Geometry: final body of the model. Coordinates: model frame, mm. A direction names the side the tool comes from. Give positions to 0.01 mm unless a question says otherwise; leave off trailing zeros. Write each loop counter-clockwise with the first axis right and the second up, starting at its lowest first coordinate (ties: lowest second). Pieces come first, ordered by that corner, then holes. Notation, with made-up numbers: M 58,-16.75 L 113,-16.75 A21 cw 113,3.25 Z; hole C 74,-12 d8. An arc over 180 degrees is marked long. Use a Markdown table: item, result. Add a question column.
1) Set-up query: faces 4 (the flat face through (0, -3, 33)), 5 (the flat face through (-31, -18, 0)), 6 (the flat face through (0, -18, -31)), 7 (the cylindrical face through (0.621, -6.386, -13.503)), 8 (the cylindrical face through (21.31, -13.32, 24.84)). Return all of +Z, -Z, +X, -X, +Y, -Y with unobstructed straight access to the full face (end or side cutting, diameter ignored); none if empty.
2) Line query: line 1 (X direction, y = -19.5, z = -20); line 2 (X direction, y = -3, z = -20); line 3 (Z direction, x = 0, y = -0.75). Output: solid intervals per line, ascending.
3) Draft query along Z for faces 1 (the flat face through (0, -3, -33)), 2 (the flat face through (34, 1, 0)), 3 (the flat face through (20, -16, 15)). Return one class per face: +Z half, -Z half, draft (parallel to the pull), parting line (faces both ways), or undercut.
4) Section C-C on x = -10. Return the cut outline in (y, z).
5) Section A-A on y = -9.5. State how many separate pieces and enclosed holes the cut face has, then the cut area to 3 significant figures.
6) Pin query (flat end, axial travel): pin 1 (12 mm diameter, centred on x = -8.5, z = -2, fed in from +Y); pin 2 (3 mm diameter, centred on x = 8, y = -6, fed in from -Z); pin 3 (2 mm diameter, centred on x = -5, y = -15.5, fed in from +Z). Return the tip coordinate at first contact, or that it passes through.
Solid Edge part; units mm, degrees
sketch "Sketch1" plane through (0, 0, 0) normal (0, -1, 0) x (1, 0, 0)
  line L0 (-34, 34) -> (34, 34)
  line L1 (34, 34) -> (34, -34)
  line L2 (34, -34) -> (-34, -34)
  line L3 (-34, -34) -> (-34, 34)
  dimension "D1" = 34
  dimension "D2" = 34
extrude "Protrusion1" add sketch "Sketch1" along normal mid plane 8
sketch "Sketch2" plane through (0, -4, 0) normal (0, -1, 0) x (1, 0, 0)
  line L0 (-31, 31) -> (31, 31)
  line L1 (31, 31) -> (31, -31)
  line L2 (31, -31) -> (-31, -31)
  line L3 (-31, -31) -> (-31, 31)
  dimension "D1" = 31
  dimension "D2" = 31
extrude "Ausprägung_2" add sketch "Sketch2" along normal blind 30
chamfer "Fase_1" distance 2 angle 45 4 edges at (0, -4, -34) (34, -4, 0) (0, -4, 34) (-34, -4, 0)
chamfer "Fase_2" distance 1 angle 45 4 edges at (-31, -34, 0) (0, -34, 31) (31, -34, 0) (0, -34, -31)
chamfer "Fase_3" distance 1 angle 45 8 edges at (31, -18.5, -31) (31, -18.5, 31) (-31, -18.5, 31) (-31, -18.5, -31) (-34, 1, -34) (34, 1, 34) (34, 1, -34) (-34, 1, 34)
hole "Bohrung_1" at (20, 4, -20) direction (0, -1, 0) diameter 8.5 end up to next
hole "Hole1" at (0, 4, 20) direction (0, -1, 0) diameter 8.5 end up to next
hole "Hole2" at (-20, 4, -20) direction (0, -1, 0) diameter 8.5 end up to next
chamfer "Fase_4" distance 1 angle 45 6 edges at (-20, -34, -24.25) (0, -34, 15.75) (20, -34, -24.25) (-24.25, 4, -20) (-4.25, 4, 20) (15.75, 4, -20)
hole "Bohrung_4" at (-20, 4, 15) direction (0, -1, 0) diameter 3.242 depth 20
hole "Hole3" at (20, 4, 14.6635) direction (0, -1, 0) diameter 3.242 depth 20
hole "Hole4" at (0, 4, -15) direction (0, -1, 0) diameter 3.242 depth 20
chamfer "Fase_5" distance 0.5 angle 45 3 edges at (0, 4, -16.621) (-20, 4, 13.379) (20, 4, 13.0425)
hole "Bohrung_11" at (-23, -34, 23) direction (0, 1, 0) diameter 5 depth 38 countersink diameter 10 countersink angle 82
hole "Hole5" at (23, -34, 23) direction (0, 1, 0) diameter 5 depth 38 countersink diameter 10 countersink angle 82
hole "Hole6" at (0, -34, -23) direction (0, 1, 0) diameter 5 depth 38 countersink diameter 10 countersink angle 82
sketch "Sketch3" plane through (0, 4, 0) normal (0, 1, 0) x (1, 0, 0)
  line L0 (-25, 10) -> (25, 10)
  line L1 (25, 10) -> (25, -10)
  line L2 (25, -10) -> (-25, -10)
  line L3 (-25, -10) -> (-25, 10)
  dimension "D1" = 25
  dimension "D2" = 25
extrude "Ausschnitt_1" cut sketch "Sketch3" against normal blind 23
fillet "Verrundung_1" radius 10 4 edges at (-25, -7.5, -10) (-25, -7.5, 10) (25, -7.5, 10) (25, -7.5, -10)
properties material "Aluminium, 1060"
Found:
| question | item | result |
|---|---|---|
| 1 | face 4 | +Z, +X, -X, -Y |
| 1 | face 5 | +Z, -Z, -X, -Y |
| 1 | face 6 | -Z, +X, -X, -Y |
| 1 | face 7 | +Y |
| 1 | face 8 | +Y, -Y |
| 2 | line 1 | -31 to -24.25, -15.75 to 15.75, 24.25 to 31 |
| 2 | line 2 | -33 to -24.25, -15.75 to 15.75, 24.25 to 33 |
| 2 | line 3 | -34 to -25.5, -20.5 to -16.62, -13.38 to -10, 10 to 15.75, 24.25 to 34 |
| 3 | face 1 | -Z half |
| 3 | face 2 | draft |
| 3 | face 3 | undercut |
| 4 | outline | M -34,-30 L -33,-31 L -4,-31 L -4,-32 L -2,-34 L 4,-34 L 4,-10 L -19,-10 L -19,10 L 4,10 L 4,34 L -2,34 L -4,32 L -4,31 L -33,31 L -34,30 Z |
| 5 | separate pieces | 1 |
| 5 | enclosed holes | 10 |
| 5 | area | 2,670 mm² |
| 6 | pin 1 | y = -19 |
| 6 | pin 2 | z = -31 |
| 6 | pin 3 | z = 31 |
